Geometry: final body of the model. Coordinates: model frame, mm. A direction names the side the tool comes from. Coordinates: 2 decimals unless noted, no trailing zeros. Order: outer loops, then holes, each group sorted by start corner. A loop starts at its lowest first (then second) coordinate and runs counter-clockwise, first axis right, second up. Notation, with made-up numbers: (-28, -5.5) - (-15, -5.5) arc R29 cw to (-15, 14.5) - close; hole circle Ø10 at (-21, -2.5). An arc over 180 degrees is marked (long way). Use a Markdown table: item, result. Add a question column.
```python
from build123d import *

# Parameters (mm, degrees)
BOSS_EXTRU_1_DEPTH           = 10
ESQUISSE4_W                  = 25
ESQUISSE4_H                  = 2.8
BOSS_EXTRU_2_DEPTH           = 1
ESQUISSE2_R                  = 1.5
ENL_V_MAT_EXTRU_1_DEPTH      = 34.421549934
ENL_V_MAT_EXTRU_1_DEPTH_BACK = 34.421549934
ESQUISSE5_W                  = 2.9
ESQUISSE5_H                  = 25
BOSS_EXTRU_3_DEPTH           = 1
ESQUISSE3_R                  = 1.5
ENL_V_MAT_EXTRU_2_DEPTH      = 34.421549934
ENL_V_MAT_EXTRU_2_DEPTH_BACK = 34.421549934


with BuildPart() as part:
    # Esquisse1 → Boss.-Extru.1 (new body)
    with BuildSketch(Plane.XY):
        with BuildLine():
            Line((-25, 0), (0, 0))
            Line((0, 0), (17.67766953, 17.67766953))
            Line((17.67766953, 17.67766953), (15.556349186, 19.798989873))
            Line((15.556349186, 19.798989873), (2.272077939, 6.514718626))
            ThreePointArc((2.272077939, 6.514718626), (-1.621002247, 3.91344561), (-6.213203436, 3))
            Line((-6.213203436, 3), (-25, 3))
            Line((-25, 3), (-25, 0))
        make_face()
    extrude(amount=BOSS_EXTRU_1_DEPTH)

    # Esquisse4 → Boss.-Extru.2 (add)
    with BuildSketch(Plane(origin=(0, 0, 0), x_dir=(-1, 0, 0), z_dir=(0, -1, 0))):
        with Locations((12.5, -5)):
            Rectangle(ESQUISSE4_W, ESQUISSE4_H)
    extrude(amount=BOSS_EXTRU_2_DEPTH)

    # Esquisse2 → Enlèv. mat.-Extru.1 (cut, two sides)
    with BuildSketch(Plane.XZ) as enl_v_mat_extru_1_sk:
        with Locations(Location((-20, 5, 0), (0, 0, 270))):
            Circle(ESQUISSE2_R)
        with Locations(Location((-10, 5, 0), (0, 0, 270))):
            Circle(ESQUISSE2_R)
    extrude(amount=ENL_V_MAT_EXTRU_1_DEPTH, mode=Mode.SUBTRACT)
    extrude(enl_v_mat_extru_1_sk.sketch, amount=-ENL_V_MAT_EXTRU_1_DEPTH_BACK, mode=Mode.SUBTRACT)

    # Esquisse5 → Boss.-Extru.3 (add)
    with BuildSketch(Plane(origin=(0, 0, 0), x_dir=(0, 0, -1), z_dir=(0.7071067811865485, -0.7071067811865466, 0))):
        with Locations((-5, 12.5)):
            Rectangle(ESQUISSE5_W, ESQUISSE5_H)
    extrude(amount=BOSS_EXTRU_3_DEPTH)

    # Esquisse3 → Enlèv. mat.-Extru.2 (cut, two sides)
    with BuildSketch(Plane(origin=(0, 0, 0), x_dir=(0, 0, -1), z_dir=(0.7071067811865485, -0.7071067811865466, 0))) as enl_v_mat_extru_2_sk:
        with Locations(Location((-5, 10, 0), (0, 0, 90))):
            Circle(ESQUISSE3_R)
        with Locations(Location((-5, 20, 0), (0, 0, 90))):
            Circle(ESQUISSE3_R)
    extrude(amount=ENL_V_MAT_EXTRU_2_DEPTH, mode=Mode.SUBTRACT)
    extrude(enl_v_mat_extru_2_sk.sketch, amount=-ENL_V_MAT_EXTRU_2_DEPTH_BACK, mode=Mode.SUBTRACT)


solid = part.part
```
1) Section query B-B (z = 2). Return the cut outline in (x, y).
2) Section query D-D (x = 9.5). Return the cut outline in (y, z).
3) Section query C-C (z = 4.5). Return the cut outline in (x, y).
4) Draft query along X for faces 1 (the cylindrical face through (-1.56, 3.94, 4.93)), 2 (the cylindrical face through (-11.464, 0.972, 5.325)), 3 (the flat face through (-2, 3, 10)). Return one class per face: released by +X, released by -X, zero draft, split by the parting line, or undercut.
5) First-contact query: pin 1 (1 mm diameter, centred on x = 5.5, z = 4, fed in from +Y); pin 2 (3 mm diameter, centred on y = 15, z = 4, fed in from +X); pin 3 (0.5 mm diameter, centred on x = -3.5, y = -0.5, fed in from -Z). Flat tips, straight axial feed; report the tip coordinate or a pass-through.
6) Section query A-A (x = -20). Return the cut outline in (y, z), and give its area (3 significant figures).
7) Access query for faces 4 (the flat face through (16.4, 15.7, 6.45)), 5 (the flat face through (9, 9, 2)), 6 (the flat face through (-14.9, -0.5, 6.4)), 7 (the flat face through (-22.7, -0.5, 3.6)). Directions: +Z, -Z, +X, -X, +Y, -Y. A direction counts if a zero-diameter tool reaches every point of the face in a straight line with its end or side. Return the directions, or none.
8) Line query: line 1 (Z direction, x = -20, y = 1.2); line 2 (Y direction, x = -19, z = 3.25); line 3 (Y direction, x = -7, z = 4). Output: solid intervals per line, ascending. Write a range as from..to.
From the geometry:
| question | item | result |
|---|---|---|
| 1 | outline | (-25, 0) - (0, 0) - (17.68, 17.68) - (15.56, 19.8) - (2.27, 6.51) arc R12 cw to (-6.21, 3) - (-25, 3) - close |
| 2 | outline | (8.09, 3.55) - (9.5, 3.55) - (9.5, 0) - (13.74, 0) - (13.74, 10) - (9.5, 10) - (9.5, 6.45) - (8.09, 6.45) - close |
| 3 | outline | (-25, -1) - (-21.41, -1) - (-21.41, 3) - (-25, 3) - close; (-18.59, -1) - (-11.41, -1) - (-11.41, 3) - (-18.59, 3) - close; (-8.59, -1) - (0, -1) - (0, 0) - (0.71, -0.71) - (6.78, 5.36) - (3.95, 8.19) - (2.27, 6.51) arc R12 cw to (-6.21, 3) - (-8.59, 3) - close; (5.95, 10.19) - (8.78, 7.36) - (13.85, 12.44) - (11.02, 15.26) - close; (13.02, 17.26) - (15.85, 14.44) - (18.38, 16.97) - (15.56, 19.8) - close |
| 4 | face 1 | released by -X |
| 4 | face 2 | undercut |
| 4 | face 3 | zero draft |
| 5 | pin 1 | stops at y = 10.24 |
| 5 | pin 2 | stops at x = 17.91 |
| 5 | pin 3 | stops at z = 3.6 |
| 6 | outline | (0, 0) - (3, 0) - (3, 3.5) - (0, 3.5) - close; (0, 6.5) - (3, 6.5) - (3, 10) - (0, 10) - close |
| 6 | area | 21.0 mm^2 |
| 7 | face 4 | +Z, +X, -Y |
| 7 | face 5 | -Z, +X, -Y |
| 7 | face 6 | +Z, -X, -Y |
| 7 | face 7 | -Z, -X, -Y |
| 8 | line 1 | z = 0..3.5, 6.5..10 |
| 8 | line 2 | y = 0..3 |
| 8 | line 3 | y = -1..3 |
